```python
from build123d import *

# Parameters (mm, degrees)
F0_W          = 76.2
F0_H          = 76.2
F0_W_2        = 69.85
F0_H_2        = 69.85
F1_DEPTH      = 454.025
F1_DEPTH_BACK = 454.025


with BuildPart() as f1:
    # F0 (on Right) → F1 (new body, two sides)
    with BuildSketch(Plane.YZ) as f1_sk:
        Rectangle(F0_W, F0_H)
        Rectangle(F0_W_2, F0_H_2, mode=Mode.SUBTRACT)
    extrude(amount=F1_DEPTH)
    extrude(f1_sk.sketch, amount=-F1_DEPTH_BACK)


solid = f1.part
```
Build history of the part. All positions in model axes, mm. A direction names the side the tool comes from. Round coordinates to 2 decimals unless told otherwise and drop trailing zeros. Loops run counter-clockwise (first coordinate to the right, second up) from the corner with the lowest first, then second, coordinate; pieces in that order, holes last.
Item 1: Pin check, flat tip, straight feed: P1, Ø8, axis at y = -1.5, z = -29, coming from the -X side. Stop position of the tip, or through.
Item 2: Saw through at A-A (x = -345.5). List the corners of the cut face in (y, z) (3 decimals).
Item 3: Drill centre line: line 1 along Z through (x, y) = (212.5, -24.5) (3 decimals). Where is it in solid material? Low to high.
Item 4: Saw through at B-B (z = 16.5). List the corners of the cut face in (x, y) (3 decimals).
Item 5: Two-plate mould, pull along Y, no slides. Class faces 3 (the face through (6, 0, 34.925)), 4 (the face through (6, -1, 38.1)), 5 (the face through (6, -38.1, -1)): released by +Y, released by -Y, zero draft, split by the parting line, or undercut.
Item 6: Which spindle directions (+Z, -Z, +X, -X, +Y, -Y) get a long thin tool onto all of the face, cutting with end or side? Do faces 1 (the face through (6, 0, -34.925)), 2 (the face through (-454.025, -3, -37)). Say none if no direction does.
Worked answers:
1. P1: passes through
2. outline: (-38.1, -38.1) - (38.1, -38.1) - (38.1, 38.1) - (-38.1, 38.1) - close; hole (-34.925, -34.925) - (34.925, -34.925) - (34.925, 34.925) - (-34.925, 34.925) - close
3. line 1: z = -38.1 to -34.925, 34.925 to 38.1
4. outline: (-454.025, -38.1) - (454.025, -38.1) - (454.025, -34.925) - (-454.025, -34.925) - close; (-454.025, 34.925) - (454.025, 34.925) - (454.025, 38.1) - (-454.025, 38.1) - close
5. face 3: undercut
5. face 4: zero draft
5. face 5: released by -Y
6. face 1: +X, -X
6. face 2: +Z, -Z, -X, +Y, -Y
